Check sheet for the modelled part. Datum: model origin and axes. Units: mm. Face numbers are marked on the shaded views. A direction names the side the tool comes from. Give positions to 0.01 mm unless a question says otherwise; leave off trailing zeros. Write each loop counter-clockwise with the first axis right and the second up, starting at its lowest first coordinate (ties: lowest second). Pieces come first, ordered by that corner, then holes. Notation, with made-up numbers: (11.5, -32) -> (44.5, -32) arc R30 ccw to (44.5, 5) -> close; hole circle Ø1 at (12, 11.5). An arc over 180 degrees is marked (long way). Answer as a JSON object with one key per item and string values.
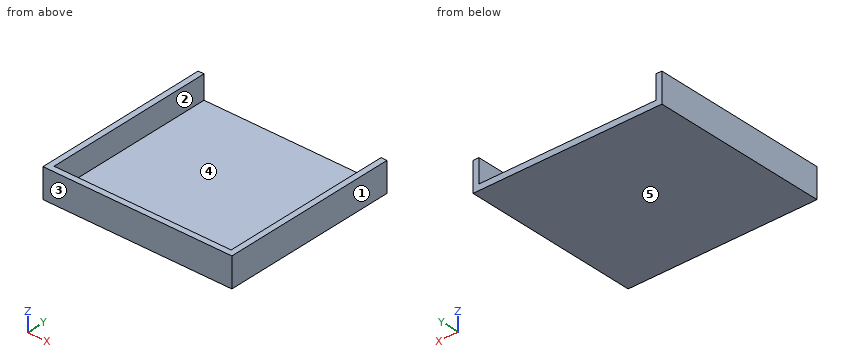
from build123d import *

# Parameters (mm, degrees)
F0_W     = 76.2
F0_H     = 2.54
F1_DEPTH = 76.2
F2_DEPTH = 76.2
F3_DEPTH = 76.2
F4_W     = 2.54
F4_H     = 10.16
F5_DEPTH = 76.2


with BuildPart() as f1:
    # F0 (on Front) → F1 (new body)
    with BuildSketch(Plane.XZ):
        with Locations((0.177208, -1.27)):
            Rectangle(F0_W, F0_H)
    extrude(amount=F1_DEPTH)

    # F0 (on Front) → F2 (join)
    with BuildSketch(Plane.XZ):
        Polygon((-37.922792, -2.54), (-37.922792, 0), (-37.922792, 10.16), (-40.462792, 10.16), (-40.462792, -2.54), align=None)
    extrude(amount=F2_DEPTH)

    # F0 (on Front) → F3 (join)
    with BuildSketch(Plane.XZ):
        Polygon((38.277208, 10.16), (38.277208, 0), (38.277208, -2.54), (40.817208, -2.54), (40.817208, 10.16), align=None)
    extrude(amount=F3_DEPTH)

    # F4 (on face) → F5 (join)
    with BuildSketch(Plane.YZ.offset(-37.922792)):
        with Locations((-74.93, 5.08)):
            Rectangle(F4_W, F4_H)
    extrude(amount=F5_DEPTH)


solid = f1.part
1. Go/stop test with flat-tipped pins: P1, Ø5, axis at x = 23.5, y = -19, coming from the +Z side; P2, Ø2, axis at x = 25, z = 5.5, coming from the +Y side. Record where each tip stops, or that it passes through.
Determined:
{"P1": "z = 0", "P2": "y = -73.66"}
2. Sectioned sample at B-B, the plane z = 3. Enter the section's corners in (x, y), plus the area to 3 significant figures.
Determined:
{"outline": "(-40.46, -76.2) -> (40.82, -76.2) -> (40.82, 0) -> (38.28, 0) -> (38.28, -73.66) -> (-37.92, -73.66) -> (-37.92, 0) -> (-40.46, 0) -> close", "area": "581 mm^2"}
3. Sectioned sample at A-A, the plane y = -39. Enter the section's corners in (x, z), plus the area to 3 significant figures.
Determined:
{"outline": "(-40.46, -2.54) -> (40.82, -2.54) -> (40.82, 10.16) -> (38.28, 10.16) -> (38.28, 0) -> (-37.92, 0) -> (-37.92, 10.16) -> (-40.46, 10.16) -> close", "area": "258 mm^2"}
4. Mould release check, pull along X, two halves, no side actions. Record for the marked faces 1, 2 and 3: released by +X, released by -X, zero draft, split by the parting line, or undercut.
Determined:
{"face 1": "released by +X", "face 2": "undercut", "face 3": "zero draft"}
5. Access from +Z, -Z, +X, -X, +Y, -Y to the whole of each face (thin tool, end or side, straight path). Record for the marked faces 4 and 5.
Determined:
{"face 4": "+Z, +Y", "face 5": "-Z, +X, -X, +Y, -Y"}
6. Sectioned sample at C-C, the plane x = -5.5. Enter the section's corners in (y, z), plus the area to 3 significant figures.
Determined:
{"outline": "(-76.2, -2.54) -> (0, -2.54) -> (0, 0) -> (-73.66, 0) -> (-73.66, 10.16) -> (-76.2, 10.16) -> close", "area": "219 mm^2"}
7. Scan lines: L1, parallel to X at y = -56, z = 6.25; L2, parallel to Y at x = 5.5, z = 5; L3, parallel to Z at x = 19.5, y = -52. Record each from-to range of solid material in increasing order. Write a range as [from, to].
Determined:
{"L1": "[-40.46, -37.92], [38.28, 40.82]", "L2": "[-76.2, -73.66]", "L3": "[-2.54, 0]"}
